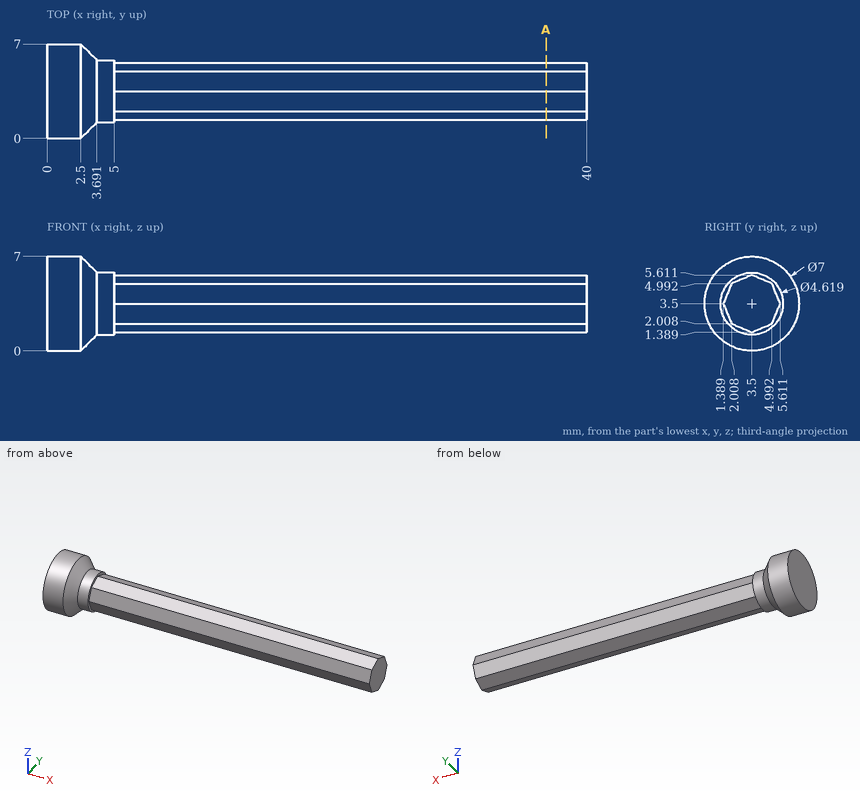
Here's the drawing with two shaded views (mm, measured from the low corner). I have some questions. Give positions to 0.01 mm unless a question says otherwise; leave off trailing zeros. Loops run counter-clockwise (first coordinate to the right, second up) from the corner with the lowest first, then second, coordinate; pieces in that order, holes last. Notation, with made-up numbers: (35.5, -15) - (56.5, -15) arc R16 cw to (56.5, -7) - close; hole circle Ø3 at (2, 5.5). An arc over 180 degrees is marked (long way). Return JSON: item names as keys, results as strings.
1. I'm going to push flat-ended pins straight in: pin 1 Ø1 at (x, y) = (4, 4.5) entering from +Z (1 decimal); pin 2 Ø3 at (x, y) = (23, 3) entering from +Z; pin 3 Ø1 at (x, y) = (6.5, 2) entering from +Z. Where does each tip first touch, or does it pass through?
Output values:
{"pin 1": "stops at z = 5.8", "pin 2": "stops at z = 5.61", "pin 3": "stops at z = 5.2"}
2. If I drill on line 1 (Y direction, x = 35.5, z = 3.5); line 2 (Z direction, x = 32, y = 3.75); line 3 (X direction, y = 1.25, z = 1.5), over which ranges is the centre line in solid material (lowest first)?
Output values:
{"line 1": "y = 1.39 to 5.61", "line 2": "z = 1.49 to 5.51", "line 3": "x = 0 to 2.99"}
3. I want a section at A-A on x = 37. Please give me the cut outline in (y, z), and give its area (3 significant figures).
Output values:
{"outline": "(1.39, 3.5) - (2.01, 2.01) - (3.5, 1.39) - (4.99, 2.01) - (5.61, 3.5) - (4.99, 4.99) - (3.5, 5.61) - (2.01, 4.99) - close", "area": "12.6 mm²"}
